Work out the finished part from the listing and answer in its coordinate system (mm). Give positions to 0.01 mm unless a question says otherwise; leave off trailing zeros. Write each loop counter-clockwise with the first axis right and the second up, starting at its lowest first coordinate (ties: lowest second). Pieces come first, ordered by that corner, then holes. Notation, with made-up numbers: (9.5, 53.25) - (35.5, 53.25) arc R32 ccw to (35.5, 86.25) - close; hole circle Ø10 at (65.25, 60.5). An arc over 180 degrees is marked (long way). Write item = value, one per line.
from build123d import *

# Parameters (mm, degrees)
F0_W     = 660.4
F0_H     = 723.9
F1_DEPTH = 12.7
F3_DEPTH = 12.701


with BuildPart() as f1:
    # F0 (on Right) → F1 (new body)
    with BuildSketch(Plane.YZ):
        with Locations((330.2, 361.95)):
            Rectangle(F0_W, F0_H)
    extrude(amount=F1_DEPTH)

    # F2 (on face) → F3 (cut, through all)
    with BuildSketch(Plane.YZ.offset(12.7)):
        with BuildLine():
            Line((508, 571.5), (152.4, 571.5))
            ThreePointArc((152.4, 571.5), (134.439488, 564.060512), (127, 546.1))
            Line((127, 546.1), (127, 190.5))
            ThreePointArc((127, 190.5), (134.439488, 172.539488), (152.4, 165.1))
            Line((152.4, 165.1), (508, 165.1))
            ThreePointArc((508, 165.1), (525.960512, 172.539488), (533.4, 190.5))
            Line((533.4, 190.5), (533.4, 546.1))
            ThreePointArc((533.4, 546.1), (525.960512, 564.060512), (508, 571.5))
        make_face()
    extrude(amount=-F3_DEPTH, mode=Mode.SUBTRACT)


solid = f1.part
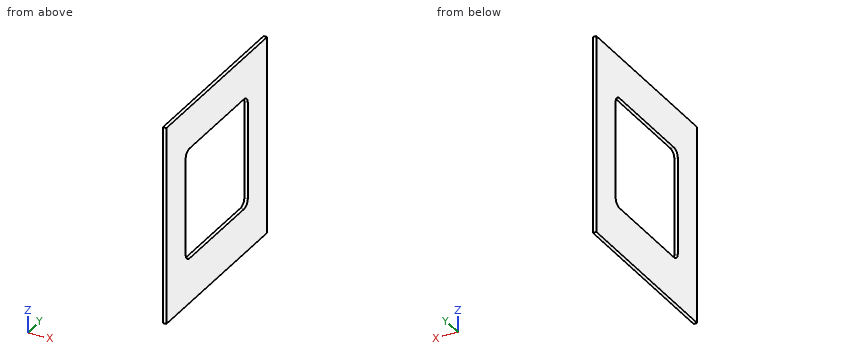
1. Find section C-C, the plane x = 9.5. Give the vertices of the cut face in (y, z).
Solution:
outline = (0, 0) - (660.4, 0) - (660.4, 723.9) - (0, 723.9) - close; hole (127, 190.5) arc R25.4 ccw to (152.4, 165.1) - (508, 165.1) arc R25.4 ccw to (533.4, 190.5) - (533.4, 546.1) arc R25.4 ccw to (508, 571.5) - (152.4, 571.5) arc R25.4 ccw to (127, 546.1) - close
2. Straight lines are drawn through the part: line 1 (Z direction, x = 3.75, y = 184); line 2 (Y direction, x = 11, z = 219); line 3 (Y direction, x = 4, z = 174). For each, find the intervals that lie inside material, in ascending order.
Solution:
line_1 = 0 to 165.1, 571.5 to 723.9
line_2 = 0 to 127, 533.4 to 660.4
line_3 = 0 to 133.09, 527.31 to 660.4
3. Find section A-A, the plane y = 367.5. Give the vertices of the cut face in (x, z).
Solution:
outline = (0, 0) - (12.7, 0) - (12.7, 165.1) - (0, 165.1) - close; (0, 571.5) - (12.7, 571.5) - (12.7, 723.9) - (0, 723.9) - close
4. Find section B-B, the plane z = 204. Give the vertices of the cut face in (x, y), then the cut area to 3 significant figures.
Solution:
outline = (0, 0) - (12.7, 0) - (12.7, 127) - (0, 127) - close; (0, 533.4) - (12.7, 533.4) - (12.7, 660.4) - (0, 660.4) - close
area = 3,230 mm^2
